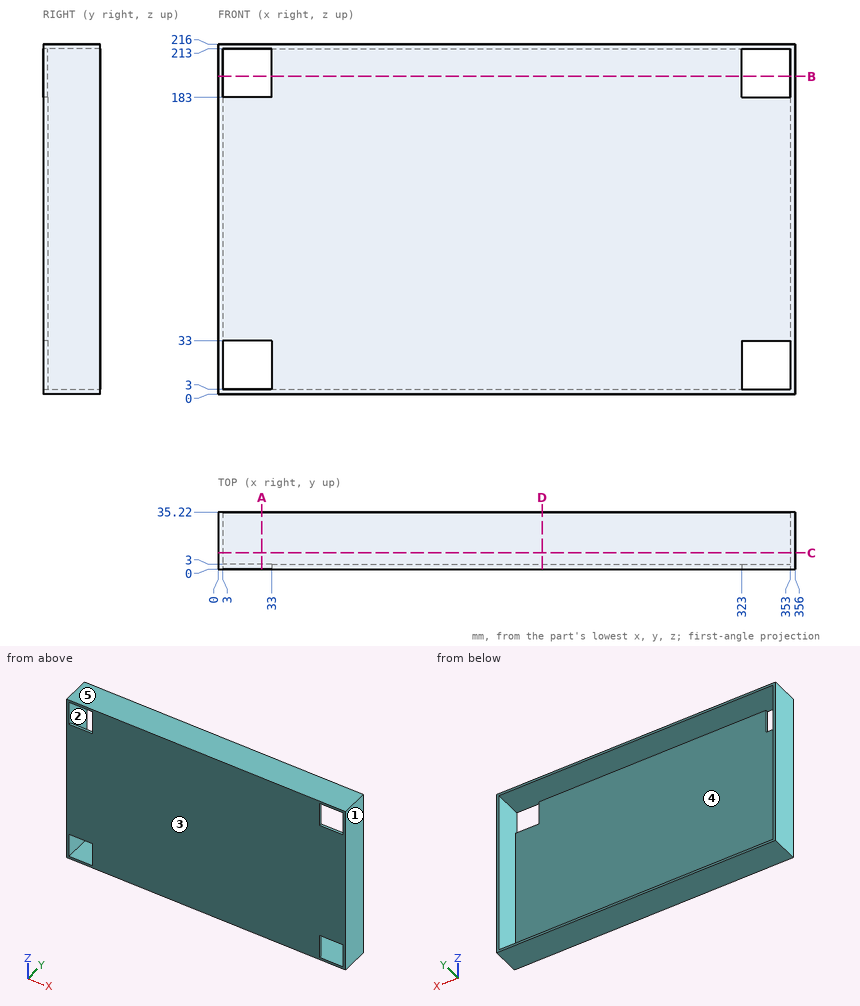
Input: dimensioned drawing with shaded views. Units: mm. Origin: part minimum x, y, z. A direction names the side the tool comes from. Round coordinates to 2 decimals unless told otherwise and drop trailing zeros. Order: outer loops, then holes, each group sorted by start corner. A loop starts at its lowest first (then second) coordinate and runs counter-clockwise, first axis right, second up. Notation, with made-up numbers: (-23.75, 1.5) - (-7.75, 1.5) arc R24 ccw to (-7.75, 38.5) - close; hole circle Ø2 at (77, 24.25). An arc over 180 degrees is marked (long way). Answer as a JSON object with one key per item and string values. Group by question number.
(1) Cut plane C-C (y = 10). Return loops of the section in (x, z), then the cut area to 3 significant figures.
(2) Cut plane D-D (x = 200). Return loops of the section in (y, z).
(3) Material intervals for probe 1 along X at (y, z) = (28.5, 12); probe 2 along Z at (x, y) = (302, 26.5); probe 3 along Y at (x, z) = (266.5, 181), sorted ascending. Write a range as from..to.
(4) Cut plane B-B (z = 196). Return loops of the section in (x, y).
(5) Cut plane A-A (x = 27). Return loops of the section in (y, z), then the cut area to 3 significant figures.
(6) Draft query along Z for the marked faces 3, 4 and 5. Return one class per face: released by +Z, released by -Z, zero draft, split by the parting line, or undercut.
(7) Pin query (flat end, axial travel): P1, Ø6, axis at y = 31.5, z = 43.5, coming from the -X side; P2, Ø6, axis at x = 137.5, z = 31.5, coming from the +Y side. Return the tip coordinate at first contact, or that it passes through.
(8) Reachability of the marked faces 1 and 2 from +Z, -Z, +X, -X, +Y, -Y: full face, straight path, thin tool, end or side. Return the list, or none.
Here are the results:
{
 "1": {"outline": "(0, 0) - (356, 0) - (356, 216) - (0, 216) - close; hole (3, 3) - (353, 3) - (353, 213) - (3, 213) - close", "area": "3,400 mm^2"},
 "2": {"outline": "(0, 0) - (35.22, 0) - (35.22, 3) - (3, 3) - (3, 213) - (35.22, 213) - (35.22, 216) - (0, 216) - close"},
 "3": {"probe 1": "x = 0..3, 353..356", "probe 2": "z = 0..3, 213..216", "probe 3": "y = 0..3"},
 "4": {"outline": "(0, 0) - (3, 0) - (3, 35.22) - (0, 35.22) - close; (33, 0) - (323, 0) - (323, 3) - (33, 3) - close; (353, 0) - (356, 0) - (356, 35.22) - (353, 35.22) - close"},
 "5": {"outline": "(0, 0) - (35.22, 0) - (35.22, 3) - (0, 3) - close; (0, 33) - (3, 33) - (3, 183) - (0, 183) - close; (0, 213) - (35.22, 213) - (35.22, 216) - (0, 216) - close", "area": "661 mm^2"},
 "6": {"face 3": "zero draft", "face 4": "undercut", "face 5": "released by +Z"},
 "7": {"P1": "stops at x = 0", "P2": "stops at y = 3"},
 "8": {"face 1": "+Z, -Z, +X, +Y, -Y", "face 2": "+Y"}
}
